Here's how the part is built. I have some questions about the finished solid (model axes, mm). Face numbers are marked on the shaded views. A direction names the side the tool comes from. Round coordinates to 2 decimals unless told otherwise and drop trailing zeros. Order: outer loops, then holes, each group sorted by start corner. A loop starts at its lowest first (then second) coordinate and runs counter-clockwise, first axis right, second up. Notation, with made-up numbers: M 38.25,-3 L 70.25,-3 A22 cw 70.25,29 Z; hole C 45,49 d2. An arc over 180 degrees is marked long. Write item = value, one per line. Start each with the question number.
Item 1: I'm going to push a flat-ended pin straight in: P1, Ø4, axis at x = -26.75, z = -5, coming from the +Y side. Where does the tip first touch, or does it pass through?
Item 2: Please list where these lines run through material, in increasing order: L1, parallel to X at y = 1.7, z = -5; L2, parallel to Z at x = -26.75, y = 2.25; L3, parallel to Z at x = -25, y = 2.1.
Item 3: We'd pull the mould along X, two halves only. Please class the marked faces 1, 2 and 3: pulls with the +X half, pulls with the -X half, needs draft (parallel to the pull), parting line crosses it, or undercut.
Item 4: For the marked faces 4 and 5, which set-ups out of +Z, -Z, +X, -X, +Y, -Y let a thin tool reach every point of the face, with its end or its side?
Item 5: I want a section at B-B, the plane z = -3. List the corners of the cut face in (x, y) for me, plus the area to 3 significant figures.
Item 6: I want a section at A-A, the plane y = 3.25. State how many separate pieces and enclosed holes the cut face has, plus the area to 3 significant figures.
Item 7: I want a section at C-C, the plane z = -8.75. List the corners of the cut face in (x, y) for me, plus the area to 3 significant figures.
Item 8: I want a section at D-D, the plane z = -1.75. List the corners of the cut face in (x, y) for me, plus the area to 3 significant figures.
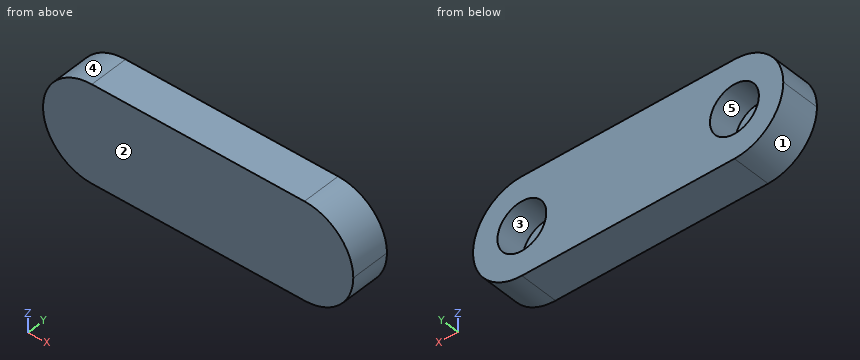
Autodesk Inventor part; units mm, degrees
ref_plane "YZ Plane" through (0, 0, 0) normal (1, 0, 0) x (0, 1, 0)
ref_plane "XZ Plane" through (0, 0, 0) normal (0, 1, 0) x (-1, 0, 0)
ref_plane "XY Plane" through (0, 0, 0) normal (0, 0, 1) x (1, 0, 0)
sketch "Sketch1" plane through (0, 0, 0) normal (0, 1, 0) x (-1, 0, 0)
  line L0 (0, 0) -> (31.75, 0)
  line L1 (31.75, 0) -> (31.75, -10)
  line L2 (31.75, -10) -> (0, -10)
  line L3 (0, -10) -> (0, 0)
  dimension "d0" = 31.75
  dimension "d1" = 10
extrude "Extrusion1" add sketch "Sketch1" along normal blind 4
sketch "Sketch2" plane through (0, 4, 0) normal (0, 1, 0) x (1, 0, 0)
  circle A0 centre (-26.75, 5) radius 2.5
  circle A1 centre (-5, 5) radius 2.5
  line L0 (-31.75, 10) -> (-31.75, 0)
  point P0 (0, 0)
  dimension "d4" = 5
  dimension "d5" = 5
  dimension "d6" = 5
  dimension "d7" = 5
  dimension "d8" = 5
extrude "Extrusion2" cut sketch "Sketch2" against normal blind 3
fillet "Fillet1" radius 5 4 edges at (-31.75, 2, 0) (0, 2, 0) (0, 2, -10) (-31.75, 2, -10)
properties part number "Linkage" material "Aluminum 6061"
Filled in:
q1.P1 = 1
q2.L1 = -31.75 to -29.25, -24.25 to -7.5, -2.5 to 0
q2.L2 = -10 to -7.5, -2.5 to 0
q2.L3 = -10 to -6.79, -3.21 to 0
q3.face_1 = pulls with the -X half
q3.face_2 = needs draft
q3.face_3 = undercut
q4.face_4 = +Z, -X, +Y, -Y
q4.face_5 = +Y
q5.outline = M -31.33,0 L -0.42,0 L -0.42,4 L -3.5,4 L -3.5,1 L -6.5,1 L -6.5,4 L -25.25,4 L -25.25,1 L -28.25,1 L -28.25,4 L -31.33,4 Z
q5.area = 106 mm^2
q6.separate_pieces = 1
q6.enclosed_holes = 2
q6.area = 257 mm^2
q7.outline = M -30.06,0 L -1.69,0 L -1.69,4 L -30.06,4 Z
q7.area = 113 mm^2
q8.outline = M -30.55,0 L -1.2,0 L -1.2,4 L -30.55,4 Z
q8.area = 117 mm^2
